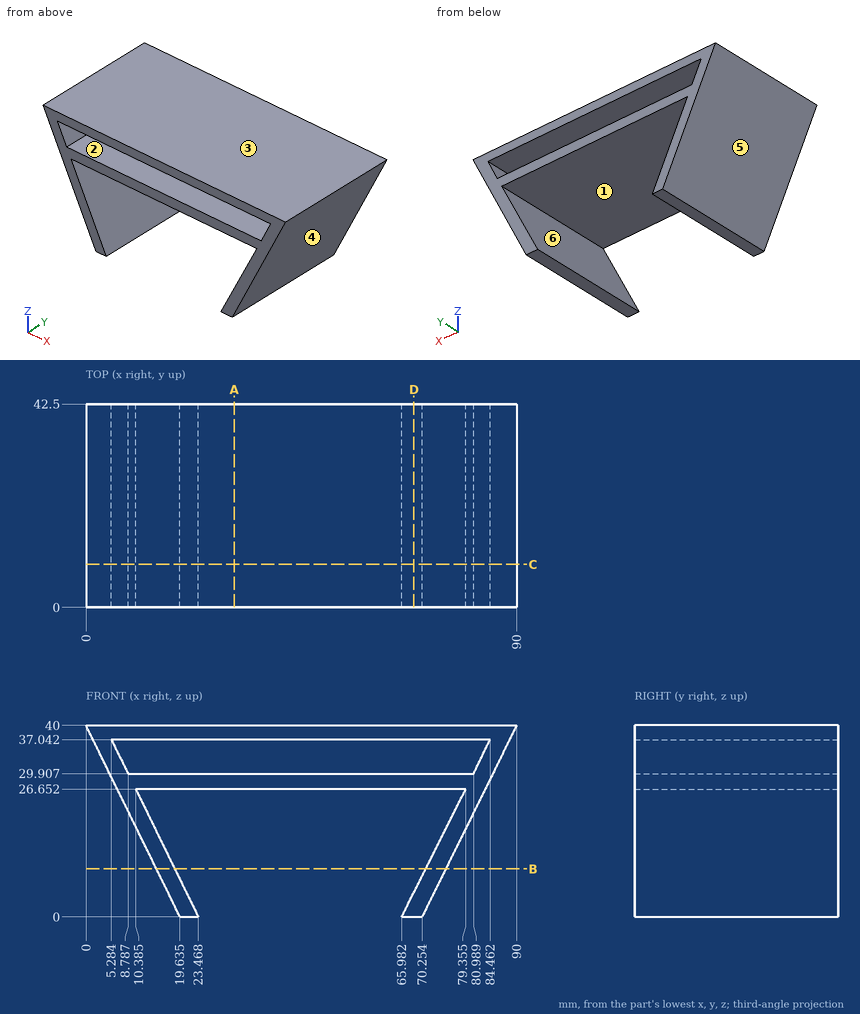
Job drawing, mm, ordinate dimensions from the low corner. One solid piece. A direction names the side the tool comes from. Round coordinates to 2 decimals unless told otherwise and drop trailing zeros. Order: outer loops, then holes, each group sorted by start corner. A loop starts at its lowest first (then second) coordinate and runs counter-clockwise, first axis right, second up. Notation, with made-up numbers: (-24, 9) - (28, 9) arc R24 ccw to (28, 41) - close; hole circle Ø11 at (-19.75, 18.5). An arc over 180 degrees is marked (long way). Use CSV: the item, a comma, the result in double quotes. Start each with the question number.
1) Saw through at A-A (x = 31). List the corners of the cut face in (y, z), and give its area (3 significant figures).
2) Two-plate mould, pull along Z, no slides. Class the marked faces 1, 2, 3 and 4: pulls with the +Z half, pulls with the -Z half, needs draft (parallel to the pull), parting line crosses it, or undercut.
3) Pin check, flat tips, straight feed: pin 1 Ø12 at (x, z) = (70, 10) entering from +Y; pin 2 Ø1 at (y, z) = (33, 9.5) entering from -X; pin 3 Ø5 at (x, y) = (14, 11.5) entering from -Z (1 decimal); pin 4 Ø4 at (x, z) = (19.5, 34) entering from +Y. Stop position of each tip, or through.
4) Saw through at D-D (x = 68.5). List the corners of the cut face in (y, z).
5) Saw through at C-C (y = 9). List the corners of the cut face in (x, z) (1 decimal).
6) Tool access for the marked faces 5 and 6: list every direction of +Z, -Z, +X, -X, +Y, -Y with a clear straight run to the whole face (end or side of a thin tool).
7) Saw through at B-B (z = 10). List the corners of the cut face in (x, y).
8) Wall check: L1, parallel to Z at x = 53, y = 27.5; L2, parallel to X at y = 21, z = 19 (1 decimal); L3, parallel to X at y = 13, z = 34 (1 decimal). Give the ranges that are in metal, low to high. Write a range as [from, to].
Values follow:
1,outline,"(0, 26.65) - (42.5, 26.65) - (42.5, 29.91) - (0, 29.91) - close; (0, 37.04) - (42.5, 37.04) - (42.5, 40) - (0, 40) - close"
1,area,"264 mm2"
2,face 1,"undercut"
2,face 2,"undercut"
2,face 3,"pulls with the +Z half"
2,face 4,"pulls with the -Z half"
3,pin 1,"stops at y = 42.5"
3,pin 2,"stops at x = 14.73"
3,pin 3,"stops at z = 6.4"
3,pin 4,"passes through"
4,outline,"(0, 0) - (42.5, 0) - (42.5, 5.02) - (0, 5.02) - close; (0, 26.65) - (42.5, 26.65) - (42.5, 29.91) - (0, 29.91) - close; (0, 37.04) - (42.5, 37.04) - (42.5, 40) - (0, 40) - close"
5,outline,"(0, 40) - (19.6, 0) - (23.5, 0) - (10.4, 26.7) - (79.4, 26.7) - (66, 0) - (70.3, 0) - (90, 40) - close; hole (5.3, 37) - (8.8, 29.9) - (81, 29.9) - (84.5, 37) - close"
6,face 5,"-Z, -X, +Y, -Y"
6,face 6,"+Y, -Y"
7,outline,"(14.73, 0) - (18.56, 0) - (18.56, 42.5) - (14.73, 42.5) - close; (71, 0) - (75.19, 0) - (75.19, 42.5) - (71, 42.5) - close"
8,L1,"z = [26.65, 29.91], [37.04, 40]"
8,L2,"x = [10.3, 14.1], [75.5, 79.6]"
8,L3,"x = [2.9, 6.8], [83, 87]"
